Could you check a few things on this model? Use its own coordinates, in mm. Face numbers are marked on the shaded views. Coordinates: 2 decimals unless noted, no trailing zeros. Write each loop counter-clockwise with the first axis right and the second up, starting at its lowest first coordinate (ties: lowest second). Pieces come first, ordered by that corner, then holes.
Item 1: If I drill on probe 1 along Z at (x, y) = (-2.5, 24.5); probe 2 along X at (y, z) = (81.5, 29.5); probe 3 along X at (y, z) = (52, 34), over which ranges is the centre line in solid material (lowest first)?
Item 2: For P1, Ø6, axis at y = 40.5, z = 23.5, coming from the -X side; P2, Ø12, axis at x = 0, z = 0, coming from the +Y side; P3, Ø5, axis at x = -21.5, y = 85.5, coming from the +Z side; P4, Ø1.5, axis at y = 37, z = -39.5, coming from the -X side (3 decimals), each with a flat end and sliding along its axis, tell me the tip position at first contact or that it passes through.
Item 3: I want a section at A-A on y = 60. State how many separate pieces and enclosed holes the cut face has, then the cut area to 3 significant figures.
Item 4: I want a section at B-B on x = 17. Please give me the cut outline in (y, z), then the cut area to 3 significant figures.
Item 5: Thinking about a two-plate mould opening in X: for the marked faces 1, 2 and 3, which applies, +X half, -X half, draft (parallel to the pull), parting line (faces both ways), or undercut?
from build123d import *

# Parameters (mm, degrees)
LOFT1_OUTLINE_W    = 80
LOFT1_OUTLINE_H    = 80
LOFT1_DEPTH        = 100
LOFT1_DRAFT        = 5.7105931
SKETCH4_R          = 7.5
CUT_EXTRUDE1_DEPTH = 123.474487085
SKETCH7_R          = 5
SKETCH9_R          = 5


# Read off the part's stored shape, not the designer's step: Loft1
with BuildPart() as part:
    # Loft1 outline → Loft1 (with draft: the straight prism first)
    with BuildSketch(Plane(origin=(0, 100, 0), x_dir=(1, 0, 0), z_dir=(0, 1, 0))):
        Rectangle(LOFT1_OUTLINE_W, LOFT1_OUTLINE_H)
    extrude(amount=-LOFT1_DEPTH)
    # Loft1: the draft: its side faces are tilted about the plane it starts from
    loft1_sides = [part.faces().sort_by_distance(p)[0] for p in [
        (40, 50, 0),
        (0, 50, -40),
        (-40, 50, 0),
        (0, 50, 40),
    ]]
    draft(loft1_sides, Plane(origin=(0, 100, 0), x_dir=(1, 0, 0), z_dir=(0, 1, 0)), LOFT1_DRAFT)

    # Sketch4 → Cut-Extrude1 (cut, through all)
    with BuildSketch(Plane(origin=(0, 100, 0), x_dir=(1, 0, 0), z_dir=(0, 1, 0))):
        with Locations(Location((0, 0, 0), (0, 0, 270))):
            Circle(SKETCH4_R)
    extrude(amount=-CUT_EXTRUDE1_DEPTH, mode=Mode.SUBTRACT)

    # Cut-Sweep1: sweep along a path in Sketch8
    with BuildLine(Plane.XY) as cut_sweep1_path:
        Line((-30, 100), (-40, 0))
    # Sketch7 → Cut-Sweep1 (sweep, cut)
    with BuildSketch(Plane(origin=(0, 100, 0), x_dir=(1, 0, 0), z_dir=(0, 1, 0))):
        with Locations((-30, 0)):
            Circle(SKETCH7_R)
    cut_sweep1 = sweep(path=cut_sweep1_path.line, mode=Mode.SUBTRACT)

    # Mirror1: Cut-Sweep1 across plane
    add(cut_sweep1.mirror(Plane(origin=(0, 0, 0), x_dir=(0, 0, 1), z_dir=(1, 0, 0))), mode=Mode.SUBTRACT)

    # Cut-Sweep2: sweep along a path in Sketch10
    with BuildLine(Plane(origin=(0, 0, 0), x_dir=(0, 0, -1), z_dir=(1, 0, 0))) as cut_sweep2_path:
        Line((-30, 100), (-40, 0))
    # Sketch9 → Cut-Sweep2 (sweep, cut)
    with BuildSketch(Plane(origin=(0, 100, 0), x_dir=(1, 0, 0), z_dir=(0, 1, 0))):
        with Locations((0, -30)):
            Circle(SKETCH9_R)
    cut_sweep2 = sweep(path=cut_sweep2_path.line, mode=Mode.SUBTRACT)

    # Mirror2: Cut-Sweep2 across plane
    add(cut_sweep2.mirror(Plane.XY), mode=Mode.SUBTRACT)


solid = part.part
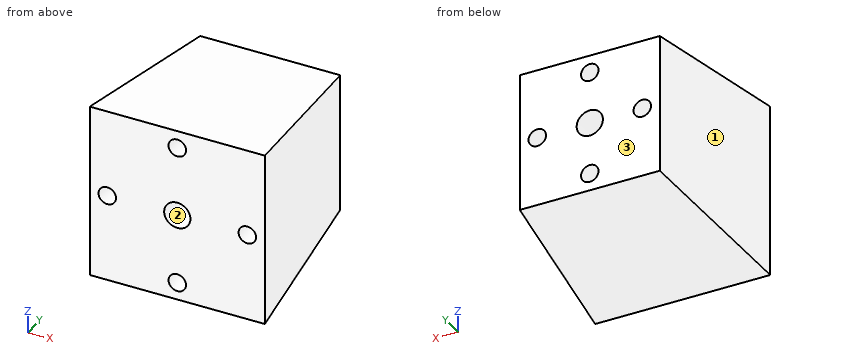
Response values:
1. probe 1: z = -47.55 to -41.88, -33.22 to -7.07, 7.07 to 33.22, 41.88 to 47.55
1. probe 2: x = -41.85 to -4.41, 4.41 to 41.85
1. probe 3: x = -44.8 to -4.94, 4.94 to 44.8
2. P1: stops at x = -46.25
2. P2: passes through
2. P3: stops at z = 41.7
2. P4: stops at x = -46.375
3. separate pieces: 1
3. enclosed holes: 5
3. area: 7,250 mm2
4. outline: (0, -50) - (100, -40) - (100, 40) - (0, 50) - close
4. area: 9,000 mm2
5. face 1: -X half
5. face 2: undercut
5. face 3: draft
